Study the drawing (mm; zero at the part's minimum x, y, z) and answer. Coordinates: 2 decimals unless noted, no trailing zeros. Order: outer loops, then holes, each group sorted by start corner. A loop starts at its lowest first (then second) coordinate and runs counter-clockwise, first axis right, second up.
1. The part is cut by section D-D, the plane z = 58. Give the vertices of the cut face in (x, y) (1 decimal).
2. The part is cut by section A-A, the plane z = 38.1. Give the vertices of the cut face in (x, y) (1 decimal).
3. The part is cut by section C-C, the plane y = 4.75. Count the separate pieces of the cut face and the enclosed holes in it.
4. Flat-ended cylindrical pins translate along their axes: pin 1 Ø6.5 at (x, z) = (16, 44.5) entering from +Y; pin 2 Ø2 at (y, z) = (5, 9.5) entering from -X; pin 3 Ø3 at (x, z) = (21.5, 22.5) entering from -Y (1 decimal); pin 4 Ø1 at (x, y) = (24, 2) entering from +Z. Find the tip coordinate at first contact, or state that the pin passes through.
5. Find the intervals of material crossed by probe 1 along Z at (x, y) = (24.25, 5.5); probe 2 along Y at (x, z) = (13.5, 62) (1 decimal); probe 3 along Y at (x, z) = (25, 56), in increasing order.
6. The part is cut by section B-B, the plane x = 25.4. Give the vertices of the cut face in (y, z).
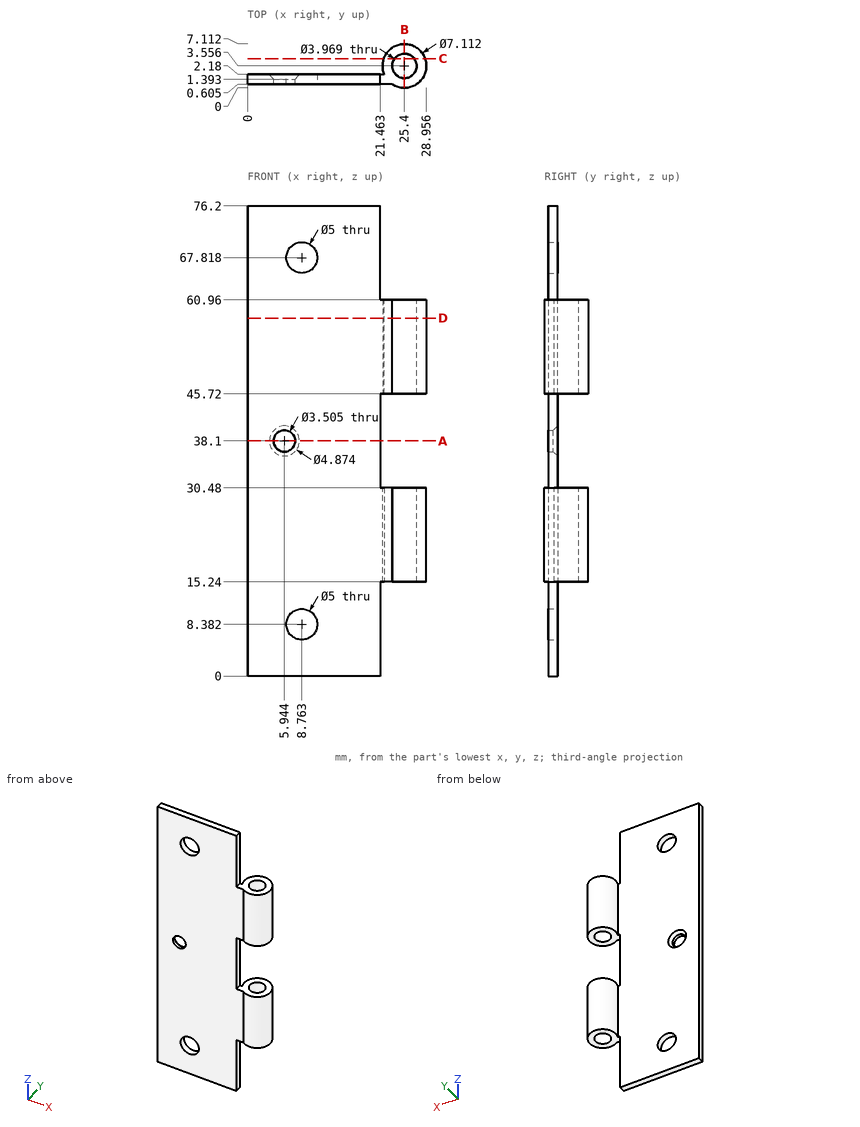
Geometry says:
1. outline: (0, 0.6) - (23.4, 0.6) arc R3.6 ccw (long way) to (22.1, 2.2) - (0, 2.2) - close; hole circle Ø4 at (25.4, 3.6)
2. outline: (0, 0.6) - (4.2, 0.6) - (4.2, 1.4) - (3.5, 2.2) - (0, 2.2) - close; (7.7, 0.6) - (21.5, 0.6) - (21.5, 2.2) - (8.4, 2.2) - (7.7, 1.4) - close
3. separate pieces: 4
3. enclosed holes: 0
4. pin 1: stops at y = 2.18
4. pin 2: passes through
4. pin 3: stops at y = 0.6
4. pin 4: stops at z = 60.96
5. probe 1: z = 15.24 to 30.48, 45.72 to 60.96
5. probe 2: y = 0.6 to 2.2
5. probe 3: y = 0.02 to 1.61, 5.5 to 7.09
6. outline: (0, 15.24) - (1.57, 15.24) - (1.57, 30.48) - (0, 30.48) - close; (0, 45.72) - (1.57, 45.72) - (1.57, 60.96) - (0, 60.96) - close; (5.54, 15.24) - (7.11, 15.24) - (7.11, 30.48) - (5.54, 30.48) - close; (5.54, 45.72) - (7.11, 45.72) - (7.11, 60.96) - (5.54, 60.96) - close
